from build123d import *

# Parameters (mm, degrees)
F1_DEPTH  = 25
F2_W      = 220.380068
F2_H      = 103.423982
F3_DEPTH  = 49.4
F6_DEPTH  = 10
F8_DEPTH  = 25
F10_DEPTH = 10
F13_DEPTH = 31.3


with BuildPart() as f1:
    # F0 (on Front) → F1 (new body, symmetric)
    with BuildSketch(Plane.XZ):
        Polygon((18.391414, 18.535092), (-18.391414, 18.535092), (-38.391414, 18.535092), (-57.109501, 11.977759), (-71.366541, -15.086461), (-48.882552, -26.930701), (-38.391414, -11.416442), (-18.391414, -18.535092), (18.391414, -18.535092), (48.391414, -3), (73.391414, -3), (73.391414, 3), (48.391414, 3), align=None)
    extrude(amount=F1_DEPTH, both=True)

    # F2 (on face) → F3 (cut)
    with BuildSketch(Plane.XY.offset(18.535092)):
        with Locations((15.868798, -6.721016)):
            Rectangle(F2_W, F2_H)
        Polygon((-57.109501, -16.336106), (-71.366541, -25), (-71.366541, 25), (-57.109501, 16.336106), (-38.391414, 25), (18.391414, 25), (48.391414, 6.266106), (73.391414, 25), (66.329263, 0), (73.391414, -25), (48.391414, -6.266106), (18.391414, -25), (-38.391414, -25), align=None, mode=Mode.SUBTRACT)
    extrude(amount=-F3_DEPTH, mode=Mode.SUBTRACT)

    # F5 (on face) → F6 (join)
    with BuildSketch(Plane.XZ.offset(25)):
        Polygon((-14.344576, 8.269234), (-32.555006, 0), (-18.391414, -31.190934), (-0.180983, -22.9217), align=None)
    extrude(amount=F6_DEPTH)

    # F7 (on face) → F8 (cut)
    with BuildSketch(Plane.XZ.offset(25)):
        Polygon((-9.286198, -27.056317), (-32.555006, 0), (-27.678248, -47.243599), (-7.968015, -40.131658), align=None)
    extrude(amount=F8_DEPTH, mode=Mode.SUBTRACT)

    # F9 (on face) → F10 (join)
    with BuildSketch(Plane(origin=(0, 25, 0), x_dir=(-1, 0, 0), z_dir=(0, 1, 0))):
        Polygon((9.286198, -27.056317), (32.555006, 0), (14.344576, 8.269234), (0.180983, -22.9217), align=None)
    extrude(amount=F10_DEPTH)

    # F12 (on Front) → F13 (cut, symmetric)
    with BuildSketch(Plane.XZ):
        Polygon((-68.431303, -23.499304), (-68.431303, -4.601866), (-78.38802, -19.232141), align=None)
    extrude(amount=F13_DEPTH, both=True, mode=Mode.SUBTRACT)


solid = f1.part
Geometry check sheet. Reference: the model listing, model coordinates, mm. A direction names the side the tool comes from. Round coordinates to 2 decimals unless told otherwise and drop trailing zeros. Write each loop counter-clockwise with the first axis right and the second up, starting at its lowest first coordinate (ties: lowest second). Pieces come first, ordered by that corner, then holes. Notation, with made-up numbers: (46, 4.25) - (68, 4.25) arc R14 ccw to (68, 12.25) - close; hole circle Ø7 at (68, 17). An arc over 180 degrees is marked (long way). One line per item, written item: value.
1. Depth check by flat-ended pin: pin 1 Ø6 at (x, y) = (-47.5, -8.5) entering from -Z; pin 2 Ø4 at (x, z) = (2, -2.5) entering from +Y; pin 3 Ø1 at (y, z) = (-10.5, 12.5) entering from +X. Enter the tip coordinate at first touch or a pass-through.
The answers:
pin 1: stops at z = -26.93
pin 2: stops at y = 25
pin 3: stops at x = 31.01
2. Cross-section at C-C on z = -5.5. Record the boundary of the cut face in (x, y).
The answers:
outline: (-66.32, -21.93) - (-57.11, -16.34) - (-38.39, -25) - (-27.82, -25) - (-27.82, -35) - (-8.09, -35) - (-8.09, -25) - (18.39, -25) - (43.56, -9.28) - (43.56, 9.28) - (18.39, 25) - (-8.09, 25) - (-8.09, 35) - (-27.82, 35) - (-27.82, 25) - (-38.39, 25) - (-57.11, 16.34) - (-66.32, 21.93) - close
3. Scan lines: L1, parallel to Y at x = 8, z = 15.5; L2, parallel to Z at x = 5.5, y = -15.5; L3, parallel to X at y = -15, z = 0.5. Record each from-to range of solid material in increasing order.
The answers:
L1: y = -25 to 25
L2: z = -18.54 to 18.54
L3: x = -63.16 to 34.41, 60.05 to 70.57
4. Set-up check for faces 5 (the face through (-28.531, -0.35, -14.926)), 6 (the face through (-9, -25, -22)), 7 (the face through (-7.164, -29.93, -7.545)), 8 (the face through (61, 0, 3)), 9 (the face through (-47.62, -20.73, -3.88)): record each of +Z, -Z, +X, -X, +Y, -Y from which the full face is reachable in a straight line by a thin tool's end or side.
The answers:
face 5: -Z, +Y, -Y
face 6: -Z, +X, -X
face 7: +Z, +X, -Y
face 8: +Z, +X, +Y, -Y
face 9: +Z, -Z, -Y
5. Cross-section at D-D on y = 2.5. Record the boundary of the cut face in (x, z).
The answers:
outline: (-68.43, -16.63) - (-48.88, -26.93) - (-38.39, -11.42) - (-18.39, -18.54) - (18.39, -18.54) - (48.39, -3) - (67.04, -3) - (67.04, 3) - (48.39, 3) - (18.39, 18.54) - (-38.39, 18.54) - (-57.11, 11.98) - (-68.43, -9.51) - close
6. Cross-section at B-B on x = -31. Record the boundary of the cut face in (y, z), and give its area (3 significant figures).
The answers:
outline: (-35, -1.81) - (-25, -1.81) - (-25, -14.05) - (25, -14.05) - (25, -1.81) - (35, -1.81) - (35, 0.71) - (25, 0.71) - (25, 18.54) - (-25, 18.54) - (-25, 0.71) - (-35, 0.71) - close
area: 1,680 mm^2
7. Mould release check, pull along X, two halves, no side actions. Record for faces 1 (the face through (-20.758, -29.93, -13.718)), 2 (the face through (60.716, 15.502, 0.042)), 3 (the face through (-61.59, 19.06, -8.91)), 4 (the face through (-16, 35, -9)): released by +X, released by -X, zero draft, split by the parting line, or undercut.
The answers:
face 1: released by -X
face 2: undercut
face 3: undercut
face 4: zero draft
8. Cross-section at A-A on y = 12. Record the boundary of the cut face in (x, z).
The answers:
outline: (-68.43, -16.63) - (-48.88, -26.93) - (-38.39, -11.42) - (-18.39, -18.54) - (18.39, -18.54) - (39.21, -7.75) - (39.21, 7.75) - (18.39, 18.54) - (-38.39, 18.54) - (-57.11, 11.98) - (-68.43, -9.51) - close; (56.04, -3) - (69.72, -3) - (69.72, 3) - (56.04, 3) - close
